```python
from build123d import *

# Parameters (mm, degrees)
SKETCH_1_R                   = 25
SKETCH_1_R_2                 = 14
EXTRUDE_1_DEPTH              = 16
EXTRUDE_3_REACH              = 40.807
EXTRUDE_4_REACH              = 60.146
EXTRUDE_4_END_RADIUS         = 240
HOLE_WIZARD_M8_1_D           = 9
HOLE_WIZARD_M8_1_CBORE_D     = 16
HOLE_WIZARD_M8_1_CBORE_DEPTH = 11
CUT_EXTRUDE_START            = 16
SKETCH_15_R                  = 22
CUT_EXTRUDE_1_DEPTH          = 2
CUT_EXTRUDE_1_DRAFT          = -45
SKETCH_16_W                  = 1.5
SKETCH_16_H                  = 1.5
PATTERN_LINEAR_1_COUNT       = 3
PATTERN_LINEAR_1_PITCH       = 4.75


with BuildPart() as part:
    # 草图1 → 凸台-拉伸1 (new body)
    with BuildSketch(Plane(origin=(0, 0, 0), x_dir=(1, 0, 0), z_dir=(0, 1, 0))):
        with Locations(Location((0, 0, 0), (0, 0, 270))):
            Circle(SKETCH_1_R)
        with Locations(Location((0, 0, 0), (0, 0, 270))):
            Circle(SKETCH_1_R_2, mode=Mode.SUBTRACT)
    extrude(amount=EXTRUDE_1_DEPTH)

    # 凸台-拉伸3: up to this cone (the profile starts inside it)
    extrude_3_end = Plane(origin=(0, 0, 0), z_dir=(0, -1, 0)).offset(-16.408173518) * Cone(5.671e-06, 855.062315179, 150.770555353, align=(Align.CENTER, Align.CENTER, Align.MIN), mode=Mode.PRIVATE)
    # 草图1<4> → 凸台-拉伸3 (add, up to the surface)
    with BuildSketch(Plane(origin=(0, 0, 0), x_dir=(1, 0, 0), z_dir=(0, 1, 0)), mode=Mode.PRIVATE) as extrude_3_sk1:
        with BuildLine():
            Line((42.105263158, 11.275939624), (8.552631579, 23.491540883))
            ThreePointArc((8.552631579, 23.491540883), (20.479450548, 14.338483367), (25, 0))
            ThreePointArc((25, 0), (20.479450548, -14.338483367), (8.552631579, -23.491540883))
            Line((8.552631579, -23.491540883), (42.105263158, -11.275939624))
            ThreePointArc((42.105263158, -11.275939624), (44.829030594, -9.867337085), (47.10686849, -7.814406331))
            ThreePointArc((47.10686849, -7.814406331), (49.60820541, 3.041310105), (42.105263158, 11.275939624))
        make_face()
    extrude_3_tool1 = extrude(extrude_3_sk1.sketch, amount=EXTRUDE_3_REACH, mode=Mode.PRIVATE) & extrude_3_end
    add(extrude_3_tool1.solids().sort_by_distance((33.391095, 0, 0))[0])
    # 草图1<4> → 凸台-拉伸3 (add, up to the surface)
    with BuildSketch(Plane(origin=(0, 0, 0), x_dir=(1, 0, 0), z_dir=(0, 1, 0)), mode=Mode.PRIVATE) as extrude_3_sk2:
        with BuildLine():
            Line((-8.552631579, 23.491540883), (-42.105263158, 11.275939624))
            ThreePointArc((-42.105263158, 11.275939624), (-49.60820541, 3.041310105), (-47.10686849, -7.814406331))
            ThreePointArc((-47.10686849, -7.814406331), (-44.829030594, -9.867337085), (-42.105263158, -11.275939624))
            Line((-42.105263158, -11.275939624), (-8.552631579, -23.491540883))
            ThreePointArc((-8.552631579, -23.491540883), (-25, 0), (-8.552631579, 23.491540883))
        make_face()
    extrude_3_tool2 = extrude(extrude_3_sk2.sketch, amount=EXTRUDE_3_REACH, mode=Mode.PRIVATE) & extrude_3_end
    add(extrude_3_tool2.solids().sort_by_distance((-33.391095, 0, 0))[0])

    # 凸台-拉伸4: up to this cylinder (the profile starts outside it)
    extrude_4_end = Plane(origin=(0, 243, 31.3806), z_dir=(0, 0, 1)) * Cylinder(EXTRUDE_4_END_RADIUS, 601.292, mode=Mode.PRIVATE)
    # 草图1<7> → 凸台-拉伸4 (add, up to the surface)
    with BuildSketch(Plane(origin=(0, 0, 0), x_dir=(1, 0, 0), z_dir=(0, 1, 0)), mode=Mode.PRIVATE) as extrude_4_sk1:
        with BuildLine():
            ThreePointArc((-42.105263158, -11.275939624), (-44.829030594, -9.867337085), (-47.10686849, -7.814406331))
            Line((-47.10686849, -7.814406331), (-15.178114149, -45.024010552))
            ThreePointArc((-15.178114149, -45.024010552), (0, -52), (15.178114149, -45.024010552))
            Line((15.178114149, -45.024010552), (47.10686849, -7.814406331))
            ThreePointArc((47.10686849, -7.814406331), (44.829030594, -9.867337085), (42.105263158, -11.275939624))
            Line((42.105263158, -11.275939624), (8.552631579, -23.491540883))
            ThreePointArc((8.552631579, -23.491540883), (0, -25), (-8.552631579, -23.491540883))
            Line((-8.552631579, -23.491540883), (-42.105263158, -11.275939624))
        make_face()
    extrude_4_tool1 = extrude(extrude_4_sk1.sketch, amount=EXTRUDE_4_REACH, mode=Mode.PRIVATE) - extrude_4_end
    add(extrude_4_tool1.solids().sort_by_distance((0, 0, 31.3806))[0])

    # M8 六角头螺栓的柱形沉头孔1 (through all)
    with Locations(Plane(origin=(0, 16, 0), x_dir=(1, 0, 0), z_dir=(0, 1, 0))):
        with Locations((-38, 0)):
            hole_wizard_m8_1 = CounterBoreHole(HOLE_WIZARD_M8_1_D / 2, HOLE_WIZARD_M8_1_CBORE_D / 2, HOLE_WIZARD_M8_1_CBORE_DEPTH)

    # 镜向1: M8 六角头螺栓的柱形沉头孔1 across plane
    add(hole_wizard_m8_1.mirror(Plane(origin=(0, 0, 0), x_dir=(0, 0, 1), z_dir=(1, 0, 0))), mode=Mode.SUBTRACT)


with BuildPart() as cut_extrude_1_tool:
    # 草图15 → 切除-拉伸1 (with draft: the straight prism first)
    with BuildSketch(Plane(origin=(0, 0, 0), x_dir=(1, 0, 0), z_dir=(0, 1, 0)).offset(CUT_EXTRUDE_START)):
        Circle(SKETCH_15_R)
    extrude(amount=-CUT_EXTRUDE_1_DEPTH)
    # 切除-拉伸1: the draft: its side faces are tilted about the plane it starts from
    cut_extrude_1_sides = [cut_extrude_1_tool.faces().sort_by_distance(p)[0] for p in [
        (-22, 15, 0),
    ]]
    draft(cut_extrude_1_sides, Plane(origin=(0, 0, 0), x_dir=(1, 0, 0), z_dir=(0, 1, 0)).offset(CUT_EXTRUDE_START), CUT_EXTRUDE_1_DRAFT)


with BuildPart() as part_1:
    add(part.part)

    # 切除-拉伸1: cut by cut_extrude_1_tool
    add(cut_extrude_1_tool.part, mode=Mode.SUBTRACT)

    # 草图16 → 切除-旋转5 (revolve, cut)
    with BuildSketch(Plane.XY, mode=Mode.PRIVATE) as cut_revolve_5_sk:
        with Locations((14.75, 11.75)):
            Rectangle(SKETCH_16_W, SKETCH_16_H)
    cut_revolve_5 = revolve(cut_revolve_5_sk.sketch.rotate(Axis((0, 21.806549083, 0), (0, -1, 0)), 90), axis=Axis((0, 21.806549083, 0), (0, -1, 0)), mode=Mode.SUBTRACT)

    # 阵列(线性)1: 切除-旋转5 ×3
    with Locations(*[(0, -i * PATTERN_LINEAR_1_PITCH, 0) for i in range(1, PATTERN_LINEAR_1_COUNT)]):
        add(cut_revolve_5, mode=Mode.SUBTRACT)


solid = part_1.part
```
Part model, mm, in its own coordinate system. A direction names the side the tool comes from. Coordinates: 2 decimals unless noted, no trailing zeros. Order: outer loops, then holes, each group sorted by start corner. A loop starts at its lowest first (then second) coordinate and runs counter-clockwise, first axis right, second up. Notation, with made-up numbers: (21, 9.25) -> (53, 9.25) arc R29 ccw to (53, 46.25) -> close; hole circle Ø10 at (-38.75, 21.25). An arc over 180 degrees is marked (long way). Put each result on its own line as item: value. Start each with the question number.
(1) Pin check, flat tips, straight feed: pin 1 Ø4 at (y, z) = (3.5, 40) entering from -X; pin 2 Ø6 at (x, y) = (-13, 5) entering from -Z; pin 3 Ø8 at (x, y) = (-26.5, 8) entering from -Z; pin 4 Ø8 at (x, z) = (38, 0) entering from +Y. Stop position of each tip, or through.
(2) Band-saw the part on A-A (z = 0). Count the separate pieces of the cut face and the enclosed holes in it, then the cut area to 3 significant figures.
(3) Mould opens along X. For faces 6 (the face through (-29.225, 11.255, 0.167)), 7 (the face through (29.225, 11.255, -0.167)), 8 (the face through (0, 2, 52)), 9 (the face through (-15.368, 7.01, -2.018)) say: pulls with the +X half, pulls with the -X half, needs draft (parallel to the pull), parting line crosses it, or undercut.
(4) Band-saw the part on B-B (z = 34). Give the cut face in (x, y).
(5) Which spindle directions (+Z, -Z, +X, -X, +Y, -Y) get a long thin tool onto all of the face, cutting with end or side? Do faces 1 (the face through (-25.09, 5.92, -17.47)), 2 (the face through (16.896, 13.221, -18.426)), 3 (the face through (-13.67, 13.24, -3.03)), 4 (the face through (0, 3, 33)), 5 (the face through (8, 3, 12)). Say none if no direction does.
(6) Probe line 1 along X through (y, z) = (13.15, 0); line 2 along Z through (x, y) = (-38, 8.5); line 3 along Y through (x, z) = (-34.5, 4.5). List the from-to ranges inside material, lowest first. Write a range as [from, to].
Determined:
1. pin 1: stops at x = -21.21
1. pin 2: stops at z = -22.96
1. pin 3: stops at z = -18.41
1. pin 4: passes through
2. separate pieces: 4
2. enclosed holes: 0
2. area: 560 mm²
3. face 6: pulls with the -X half
3. face 7: pulls with the +X half
3. face 8: parting line crosses it
3. face 9: undercut
4. outline: (-24.64, 0) -> (24.64, 0) -> (24.64, 4.27) arc R240 cw to (-24.64, 4.27) -> close
5. face 1: -Z, -X, +Y, -Y
5. face 2: +Y
5. face 3: +Y, -Y
5. face 4: +Z, +Y
5. face 5: none
6. line 1: x = [-25, -14], [14, 25]
6. line 2: z = [-12.77, -8], [8, 12.77]
6. line 3: y = [0, 5]
